Work out the finished part from the listing and answer in its coordinate system (mm). A direction names the side the tool comes from. Give positions to 0.01 mm unless a question says otherwise; leave off trailing zeros. Order: outer loops, then holes, each group sorted by start corner. A loop starts at its lowest first (then second) coordinate and runs counter-clockwise, first axis right, second up.
Autodesk Inventor part; units mm, degrees
ref_plane "YZ Plane" through (0, 0, 0) normal (1, 0, 0) x (0, 1, 0)
ref_plane "XZ Plane" through (0, 0, 0) normal (0, 1, 0) x (-1, 0, 0)
ref_plane "XY Plane" through (0, 0, 0) normal (0, 0, 1) x (1, 0, 0)
sketch "Sketch1" plane through (0, 0, 0) normal (0, 1, 0) x (-1, 0, 0)
  circle A0 centre (0, 0) radius 11 construction
  circle A1 centre (0, 0) radius 8.5 construction
  circle A2 centre (0, -8.5) radius 1.5
  circle A3 centre (7.3612, -4.25) radius 1.5
  circle A4 centre (7.3612, 4.25) radius 1.5
  circle A5 centre (0, 8.5) radius 1.5
  circle A6 centre (-7.3612, 4.25) radius 1.5
  circle A7 centre (-7.3612, -4.25) radius 1.5
  circle A8 centre (0, 0) radius 5
  line L0 (14, 16) -> (-14, 16) construction
  line L1 (-14, 16) -> (-14, -16) construction
  line L2 (-14, -16) -> (14, -16) construction
  line L3 (14, -16) -> (14, 16) construction
  line L4 (11, 16) -> (11, -16) construction
  line L5 (14, 13) -> (-14, 13) construction
  line L6 (-11, 16) -> (-11, -16) construction
  line L7 (14, -13) -> (-14, -13) construction
  line L8 (8, 16) -> (-8, 16)
  line L9 (-8, 16) -> (-8, 13)
  line L10 (-8, 13) -> (-14, 13)
  line L11 (-14, 13) -> (-14, -13)
  line L12 (-14, -13) -> (-8, -13)
  line L13 (-8, -13) -> (-8, -16)
  line L14 (-8, -16) -> (8, -16)
  line L15 (8, -16) -> (8, -13)
  line L16 (8, -13) -> (14, -13)
  line L17 (14, 13) -> (8, 13)
  line L18 (8, 13) -> (8, 16)
  circle A9 centre (0, 0) radius 25 construction
  line L19 (14, 13) -> (14, 9)
  line L20 (14, 9) -> (17, 9)
  line L21 (17, 9) -> (17, -9)
  line L22 (17, -9) -> (14, -9)
  line L23 (14, -9) -> (14, -13)
  circle A10 centre (10, 9) radius 0.9
  circle A11 centre (-10, 9) radius 0.9
  circle A12 centre (10, -9) radius 0.9
  circle A13 centre (-10, -9) radius 0.9
  point P0 (0, -16)
  point P1 (14, 0)
  point P2 (0, 16)
  point P3 (17, 0)
  dimension "d1" = 17
  dimension "d0" = 22
  dimension "d3" = 3
  dimension "d6" = 360
  dimension "d8" = 10
  dimension "d9" = 28
  dimension "d10" = 32
  dimension "d11" = 3
  dimension "d12" = 3
  dimension "d13" = 3
  dimension "d14" = 3
  dimension "d16" = 50
  dimension "d19" = 6
  dimension "d20" = 3
  dimension "d21" = 4
  dimension "d22" = 1.8
  dimension "d23" = 4
  dimension "d24" = 4
  dimension "d25" = 1.8
  dimension "d26" = 4
  dimension "d27" = 1.8
  dimension "d28" = 4
  dimension "d29" = 1.8
extrude "Extrusion1" add sketch "Sketch1" along normal blind 3
sketch "Sketch3" plane through (0, 0, 0) normal (0, -1, 0) x (1, 0, 0)
  circle A0 centre (0, 0) radius 5
  circle A1 centre (10, -9) radius 0.9
  circle A2 centre (-10, -9) radius 0.9
  circle A3 centre (10, 9) radius 0.9
  circle A4 centre (-10, 9) radius 0.9
  circle A5 centre (7.3612, -4.25) radius 1.5
  circle A6 centre (7.3612, 4.25) radius 1.5
  circle A7 centre (0, 8.5) radius 1.5
  circle A8 centre (-7.3612, 4.25) radius 1.5
  circle A9 centre (-7.3612, -4.25) radius 1.5
  circle A10 centre (0, -8.5) radius 1.5
  line L0 (-14, 13) -> (-8, 13)
  line L1 (-14, 9) -> (-14, 13)
  line L2 (-17, 9) -> (-14, 9)
  line L3 (-17, -9) -> (-17, 9)
  line L4 (-14, -9) -> (-17, -9)
  line L5 (-14, -13) -> (-14, -9)
  line L6 (-8, -13) -> (-14, -13)
  line L7 (-8, -16) -> (-8, -13)
  line L8 (8, -16) -> (-8, -16)
  line L9 (8, -13) -> (8, -16)
  line L10 (14, -13) -> (8, -13)
  line L11 (14, 13) -> (14, -13)
  line L12 (8, 13) -> (14, 13)
  line L13 (8, 16) -> (8, 13)
  line L14 (-8, 16) -> (8, 16)
  line L15 (-8, 13) -> (-8, 16)
equation "\"d12\" = d11"
equation "\"d13\" = d11"
equation "\"d14\" = d11"
equation "\"d20\" = d11"
equation "\"d24\" = d23"
equation "\"d25\" = d22"
equation "\"d26\" = d24"
equation "\"d27\" = d22"
equation "\"d28\" = d23"
equation "\"d29\" = d22"
properties part number "motor mount" material "Polycarbonate, Clear"
1. Given P1, Ø2.5, axis at x = 0, z = -8.5, coming from the -Y side; P2, Ø0.9, axis at y = 1.5, z = 15, coming from the -X side; P3, Ø0.9, axis at x = -15.5, y = 2, coming from the +Z side, each flat-ended and moving along its own axis, determine where each tip first touches the part or whether it passes through.
Findings below:
P1: passes through
P2: stops at x = -8
P3: stops at z = 9
2. The part is cut by section A-A (x = 0). Write down the section's boundary in (y, z), then the cut area to 3 significant figures.
Findings below:
outline: (0, -16) - (3, -16) - (3, -10) - (0, -10) - close; (0, -7) - (3, -7) - (3, -5) - (0, -5) - close; (0, 5) - (3, 5) - (3, 7) - (0, 7) - close; (0, 10) - (3, 10) - (3, 16) - (0, 16) - close
area: 48.0 mm2
3. The part is cut by section D-D (z = -8.5). Write down the section's boundary in (x, y).
Findings below:
outline: (-17, 0) - (-10.75, 0) - (-10.75, 3) - (-17, 3) - close; (-9.25, 0) - (-1.5, 0) - (-1.5, 3) - (-9.25, 3) - close; (1.5, 0) - (9.25, 0) - (9.25, 3) - (1.5, 3) - close; (10.75, 0) - (14, 0) - (14, 3) - (10.75, 3) - close
4. Which of the six approach directions +Z, -Z, +X, -X, +Y, -Y give full straight-line access (tool end or side, diameter ignored) to faces 4 (the face through (8, 1, 15)), 5 (the face through (-14, 1, 11)), 6 (the face through (-16, 1, -9))?
Findings below:
face 4: +Z, +X, +Y, -Y
face 5: +Z, -X, +Y, -Y
face 6: -Z, -X, +Y, -Y
5. The part is cut by section C-C (x = 10). Write down the section's boundary in (y, z), then the cut area to 3 significant figures.
Findings below:
outline: (0, -13) - (3, -13) - (3, -9.9) - (0, -9.9) - close; (0, -8.1) - (3, -8.1) - (3, 8.1) - (0, 8.1) - close; (0, 9.9) - (3, 9.9) - (3, 13) - (0, 13) - close
area: 67.2 mm2
6. The part is cut by section B-B (y = 1.6). State how many separate pieces and enclosed holes the cut face has, then the cut area to 3 significant figures.
Findings below:
separate pieces: 1
enclosed holes: 11
area: 747 mm2
7. Straight lines are drawn through the part: probe 1 along Z at (x, y) = (-10, 0.9); probe 2 along X at (y, z) = (0.2, -3.5); probe 3 along Z at (x, y) = (-6.5, 1.05). For each, find the intervals that lie inside material, in ascending order.
Findings below:
probe 1: z = -13 to -9.9, -8.1 to 8.1, 9.9 to 13
probe 2: x = -17 to -8.66, -6.06 to -3.57, 3.57 to 6.06, 8.66 to 14
probe 3: z = -16 to -5.48, -3.02 to 3.02, 5.48 to 16
8. The mould has two halves that part along Z. Classify faces 1 (the face through (11, 1, -13)), 2 (the face through (-14, 1, -11)), 3 (the face through (-5.863, 1.479, -4.316)): pulls with the +Z half, pulls with the -Z half, needs draft (parallel to the pull), parting line crosses it, or undercut.
Findings below:
face 1: pulls with the -Z half
face 2: needs draft
face 3: undercut
